Study the drawing (mm; zero at the part's minimum x, y, z) and answer. A direction names the side the tool comes from. Coordinates: 2 decimals unless noted, no trailing zeros. Order: outer loops, then holes, each group sorted by start corner. A loop starts at its lowest first (then second) coordinate and runs counter-clockwise, first axis right, second up. Notation, with made-up numbers: (83.25, 26.25) - (139.25, 26.25) arc R24 cw to (139.25, 50.25) - close; hole circle Ø8 at (-12, -6.75). An arc over 180 degrees is marked (long way). Write item = value, one per line.
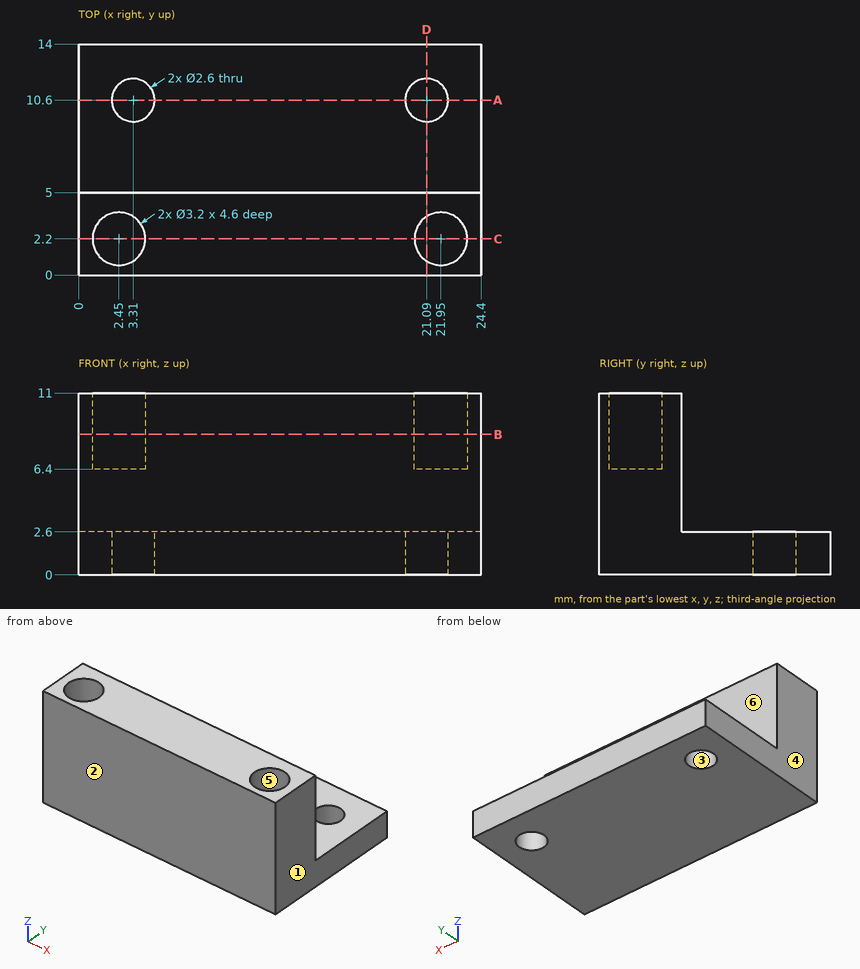
1) The part is cut by section D-D (x = 21.09). Determine the outline of the cut face in (y, z), and give its area (3 significant figures).
Returned:
outline = (0, 0) - (9.3, 0) - (9.3, 2.6) - (5, 2.6) - (5, 11) - (3.55, 11) - (3.55, 6.4) - (0.85, 6.4) - (0.85, 11) - (0, 11) - close; (11.9, 0) - (14, 0) - (14, 2.6) - (11.9, 2.6) - close
area = 59.2 mm^2
2) Flat-ended cylindrical pins translate along their axes: pin 1 Ø2.5 at (x, z) = (11.5, 7) entering from +Y; pin 2 Ø1.6 at (x, y) = (3.31, 10.6) entering from +Z; pin 3 Ø1 at (x, y) = (2, 1.5) entering from +Z. Find the tip coordinate at first contact, or state that the pin passes through.
Returned:
pin_1 = 5
pin_2 = through
pin_3 = 6.4
3) The part is cut by section A-A (y = 10.6). Determine the outline of the cut face in (x, z).
Returned:
outline = (0, 0) - (2.01, 0) - (2.01, 2.6) - (0, 2.6) - close; (4.61, 0) - (19.79, 0) - (19.79, 2.6) - (4.61, 2.6) - close; (22.39, 0) - (24.4, 0) - (24.4, 2.6) - (22.39, 2.6) - close
4) For the marked faces 4, 5 and 6, determine the directions among +Z, -Z, +X, -X, +Y, -Y from which every point of the face is accessible in a straight line to the end or side of a thin tool.
Returned:
face_4 = +Z, -Z, -X, +Y, -Y
face_5 = +Z
face_6 = +Z, +X, -X, +Y
5) The part is cut by section B-B (z = 8.5). Determine the outline of the cut face in (x, y).
Returned:
outline = (0, 0) - (24.4, 0) - (24.4, 5) - (0, 5) - close; hole circle Ø3.2 at (2.45, 2.2); hole circle Ø3.2 at (21.95, 2.2)
6) The part is cut by section C-C (y = 2.2). Determine the outline of the cut face in (x, z).
Returned:
outline = (0, 0) - (24.4, 0) - (24.4, 11) - (23.55, 11) - (23.55, 6.4) - (20.35, 6.4) - (20.35, 11) - (4.05, 11) - (4.05, 6.4) - (0.85, 6.4) - (0.85, 11) - (0, 11) - close
7) Determine the mould class of the marked faces 1, 2 and 3 for opening direction Y: pulls with the +Y half, pulls with the -Y half, needs draft (parallel to the pull), parting line crosses it, or undercut.
Returned:
face_1 = needs draft
face_2 = pulls with the -Y half
face_3 = undercut
8) Straight lines are drawn through the part: line 1 along Y through (x, z) = (21.09, 1.9); line 2 along Y through (x, z) = (2.45, 9.55); line 3 along X through (y, z) = (10.75, 2). For each, find the intervals that lie inside material, in ascending order. Write a range as from..to.
Returned:
line_1 = 0..9.3, 11.9..14
line_2 = 0..0.6, 3.8..5
line_3 = 0..2.02, 4.6..19.8, 22.38..24.4
